CAD build for the part. Positions are in the model's coordinates, mm. Coordinates: 2 decimals unless noted, no trailing zeros. Loops run counter-clockwise (first coordinate to the right, second up) from the corner with the lowest first, then second, coordinate; pieces in that order, holes last. Notation, with made-up numbers: (-2.75, 64.25) -> (52.25, 64.25) arc R17 cw to (52.25, 88.25) -> close; hole circle Ø11 at (87.25, 77.5). An arc over 180 degrees is marked (long way). Return JSON: item names as keys, results as strings. Group by question number.
(1) Probe L1, parallel to X at y = 1.55, z = 0.5 (3 decimals); L2, parallel to X at y = 1.7, z = 4.5; L3, parallel to X at y = 1.85, z = 10. List the from-to ranges inside material, lowest first.
(2) Saw through at B-B on z = 10. Write the cut outline in (x, y) (3 decimals).
(3) Saw through at A-A on z = 0. Write the cut outline in (x, y) (3 decimals), then the cut area to 3 significant figures.
(4) Saw through at C-C on y = 2. Write the cut outline in (x, z).
(5) Flat gauge pin, fed straight in: pin 1 Ø12 at (x, z) = (97, 12) entering from -Y. Where does the tip first touch, or does it go through?
(6) Saw through at D-D on z = 20.5. Write the cut outline in (x, y) (3 decimals), then the cut area to 3 significant figures.
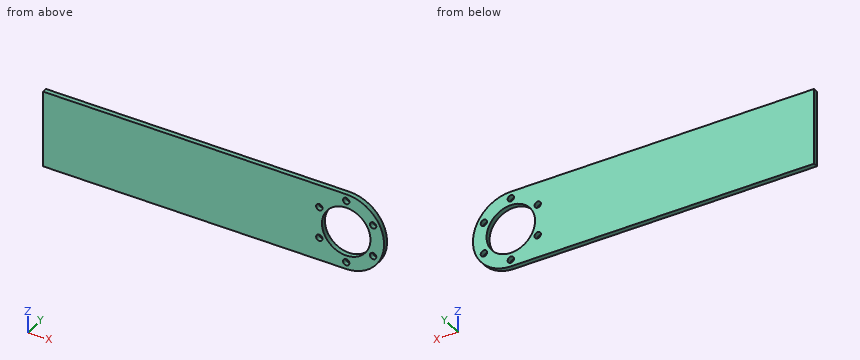
```python
from build123d import *

# Parameters (mm, degrees)
BOSS_EXTRUDE1_DEPTH = 3.175
SKETCH2_R           = 16
SKETCH2_R_2         = 2.1
CUT_EXTRUDE1_DEPTH  = 128.515021174


with BuildPart() as part:
    # Sketch1 → Boss-Extrude1 (new body)
    with BuildSketch(Plane(origin=(0, 0, 0), x_dir=(1, 0, 0), z_dir=(0, 1, 0))):
        with BuildLine():
            Line((-100, -25), (100, -25))
            ThreePointArc((100, -25), (125, 0), (100, 25))
            Line((100, 25), (-100, 25))
            Line((-100, 25), (-100, -25))
        make_face()
    extrude(amount=BOSS_EXTRUDE1_DEPTH)

    # Sketch2 → Cut-Extrude1 (cut, through all)
    with BuildSketch(Plane(origin=(0, 3.175, 0), x_dir=(1, 0, 0), z_dir=(0, 1, 0))):
        with Locations(Location((100, 0, 0), (0, 0, 270))):
            Circle(SKETCH2_R)
        with Locations(Location((100, 20.5, 0), (0, 0, 270))):
            Circle(SKETCH2_R_2)
        with Locations(Location((117.753520778, 10.25, 0), (0, 0, 270))):
            Circle(SKETCH2_R_2)
        with Locations(Location((117.753520778, -10.25, 0), (0, 0, 270))):
            Circle(SKETCH2_R_2)
        with Locations(Location((100, -20.5, 0), (0, 0, 270))):
            Circle(SKETCH2_R_2)
        with Locations(Location((82.246479222, -10.25, 0), (0, 0, 270))):
            Circle(SKETCH2_R_2)
        with Locations(Location((82.246479222, 10.25, 0), (0, 0, 270))):
            Circle(SKETCH2_R_2)
    extrude(amount=-CUT_EXTRUDE1_DEPTH, mode=Mode.SUBTRACT)


solid = part.part
```
Geometry results:
{
 "1": {"L1": "-100 to 84.008, 115.992 to 124.995", "L2": "-100 to 84.65, 115.35 to 124.59", "L3": "-100 to 80.16, 84.33 to 87.51, 112.49 to 115.67, 119.84 to 122.91"},
 "2": {"outline": "(-100, 0) -> (80.161, 0) -> (80.161, 3.175) -> (-100, 3.175) -> close; (84.332, 0) -> (87.51, 0) -> (87.51, 3.175) -> (84.332, 3.175) -> close; (112.49, 0) -> (115.668, 0) -> (115.668, 3.175) -> (112.49, 3.175) -> close; (119.839, 0) -> (122.913, 0) -> (122.913, 3.175) -> (119.839, 3.175) -> close"},
 "3": {"outline": "(-100, 0) -> (84, 0) -> (84, 3.175) -> (-100, 3.175) -> close; (116, 0) -> (125, 0) -> (125, 3.175) -> (116, 3.175) -> close", "area": "613 mm²"},
 "4": {"outline": "(-100, -25) -> (100, -25) arc R25 ccw to (100, 25) -> (-100, 25) -> close; hole circle Ø4.2 at (82.25, -10.25); hole circle Ø4.2 at (82.25, 10.25); hole circle Ø32 at (100, 0); hole circle Ø4.2 at (100, -20.5); hole circle Ø4.2 at (100, 20.5); hole circle Ø4.2 at (117.75, -10.25); hole circle Ø4.2 at (117.75, 10.25)"},
 "5": {"pin 1": "y = 0"},
 "6": {"outline": "(-100, 0) -> (97.9, 0) -> (97.9, 3.175) -> (-100, 3.175) -> close; (102.1, 0) -> (114.309, 0) -> (114.309, 3.175) -> (102.1, 3.175) -> close", "area": "667 mm²"}
}
